```python
from build123d import *

# Parameters (mm, degrees)
BOSS_EXTRUDE1_DEPTH   = 5.5
M3X0_5_TAPPED_HOLE1_D = 2.5
FILLET1_R             = 0.127


with BuildPart() as part:
    # Sketch1 → Boss-Extrude1 (new, symmetric)
    with BuildSketch(Plane(origin=(0, 0, 0), x_dir=(1, 0, 0), z_dir=(0, 1, 0))):
        Polygon((2.742298309, 0), (1.371149154, 2.3749), (-1.371149154, 2.3749), (-2.742298309, 0), (-1.371149154, -2.3749), (1.371149154, -2.3749), align=None)
    extrude(amount=BOSS_EXTRUDE1_DEPTH, both=True)

    # M3x0.5 Tapped Hole1 (through all)
    with Locations(Plane(origin=(0, 5.5, 0), x_dir=(1, 0, 0), z_dir=(0, 1, 0))):
        with Locations((0, 0)):
            Hole(M3X0_5_TAPPED_HOLE1_D / 2)

    # Fillet1
    fillet1_edges = [part.edges().sort_by_distance(p)[0] for p in [
        (0, 5.5, -2.3749),
        (-2.056723731, 5.5, -1.18745),
        (-2.056723731, 5.5, 1.18745),
        (0, 5.5, 2.3749),
        (1.25, 5.5, 0),
        (1.25, -5.5, 0),
        (2.056723731, 5.5, 1.18745),
        (0, -5.5, 2.3749),
        (-2.056723731, -5.5, 1.18745),
        (-2.056723731, -5.5, -1.18745),
        (2.056723731, 5.5, -1.18745),
        (0, -5.5, -2.3749),
        (2.056723731, -5.5, -1.18745),
        (2.056723731, -5.5, 1.18745),
    ]]
    fillet(fillet1_edges, radius=FILLET1_R)


solid = part.part
```
CAD build for the part. Positions are in the model's coordinates, mm. Give positions to 0.01 mm unless a question says otherwise; leave off trailing zeros. Loops run counter-clockwise (first coordinate to the right, second up) from the corner with the lowest first, then second, coordinate; pieces in that order, holes last. Notation, with made-up numbers: M -4,0.5 L 0,0.5 A19 ccw 0,11.5 Z; hole C 79,60.5 d7. An arc over 180 degrees is marked long. Use one line per item in the form item = value.
Item 1: Flat gauge pins, fed straight in: pin 1 (1 mm diameter, centred on y = 4.5, z = 1, fed in from +X); pin 2 (2 mm diameter, centred on x = 0, z = 0, fed in from +Y). Where does each tip first touch, or does it go through?
Determined:
pin_1 = 2.45
pin_2 = through
Item 2: Slice it at A-A (y = 2.5). List the corners of the cut face in (x, z).
Determined:
outline = M -2.74,0 L -1.37,-2.37 L 1.37,-2.37 L 2.74,0 L 1.37,2.37 L -1.37,2.37 Z; hole C 0,0 d2.5
Item 3: Slice it at B-B (x = 0). List the corners of the cut face in (y, z), plus the area to 3 significant figures.
Determined:
outline = M -5.5,-2.25 A0.13 ccw -5.37,-2.37 L 5.37,-2.37 A0.13 ccw 5.5,-2.25 L 5.5,-1.38 A0.13 ccw 5.37,-1.25 L -5.37,-1.25 A0.13 ccw -5.5,-1.38 Z; M -5.5,1.38 A0.13 ccw -5.37,1.25 L 5.37,1.25 A0.13 ccw 5.5,1.38 L 5.5,2.25 A0.13 ccw 5.37,2.37 L -5.37,2.37 A0.13 ccw -5.5,2.25 Z
area = 24.7 mm2
Item 4: Two-plate mould, pull along X, no slides. Class faces 1 (the face through (2.05, 0.08, 1.2)), 2 (the face through (0, 0, 2.375)), 3 (the face through (0.27, -0.08, 1.22)): pulls with the +X half, pulls with the -X half, needs draft (parallel to the pull), parting line crosses it, or undercut.
Determined:
face_1 = pulls with the +X half
face_2 = needs draft
face_3 = undercut
Item 5: Drill centre lines: probe 1 along Z at (x, y) = (0, 0.75); probe 2 along X at (y, z) = (-0.25, 0.25); probe 3 along X at (y, z) = (-4.5, 0.1). Where is each one in solid material? Low to high. Write a range as from..to.
Determined:
probe_1 = -2.37..-1.25, 1.25..2.37
probe_2 = -2.6..-1.22, 1.22..2.6
probe_3 = -2.68..-1.25, 1.25..2.68
